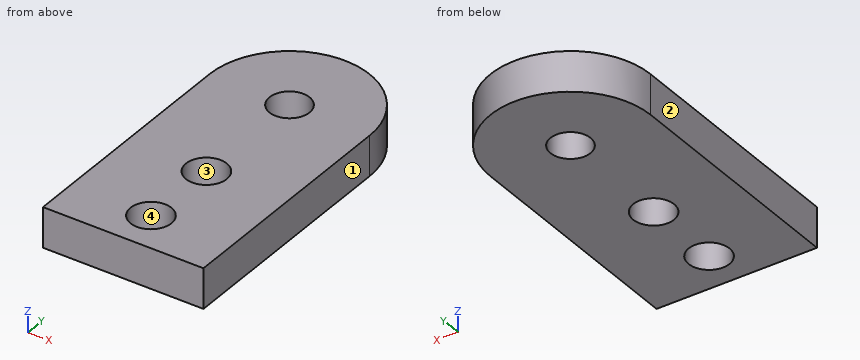
from build123d import *

# Parameters (mm, degrees)
SKETCH1_R           = 2.55
BOSS_EXTRUDE1_DEPTH = 5
SKETCH2_R           = 2.5
CUT_EXTRUDE1_DEPTH  = 5


with BuildPart() as part:
    # Sketch1 → Boss-Extrude1 (new body)
    with BuildSketch(Plane.XY):
        with BuildLine():
            Line((-10, 0), (-10, -30))
            Line((-10, -30), (10, -30))
            Line((10, -30), (10, 0))
            ThreePointArc((10, 0), (0, 10), (-10, 0))
        make_face()
        with Locations((0, -25)):
            Circle(SKETCH1_R, mode=Mode.SUBTRACT)
        with Locations((0, -15)):
            Circle(SKETCH1_R, mode=Mode.SUBTRACT)
    extrude(amount=BOSS_EXTRUDE1_DEPTH)

    # Sketch2 → Cut-Extrude1 (cut)
    with BuildSketch(Plane.XY.offset(5)):
        Circle(SKETCH2_R)
    extrude(amount=-CUT_EXTRUDE1_DEPTH, mode=Mode.SUBTRACT)


solid = part.part
The model under review builds one solid part; all positions refer to its coordinate system, in mm. Face numbers are marked on the shaded views. Give positions to 0.01 mm unless a question says otherwise; leave off trailing zeros. Order: outer loops, then holes, each group sorted by start corner. A loop starts at its lowest first (then second) coordinate and runs counter-clockwise, first axis right, second up. Notation, with made-up numbers: M 2.25,37 L 36.25,37 A17 ccw 36.25,59 Z; hole C 66.5,40 d11. An arc over 180 degrees is marked long. One line per question, with ' | ' between items. Start each with the question number.
1) Mouldability with a two-part tool opening along X and no side actions: class the marked faces 1, 2, 3 and 4 as pulls with the +X half, pulls with the -X half, needs draft (parallel to the pull), parting line crosses it, or undercut.
2) Consider section B-B, the plane y = -15. Give the boundary of the cut face in (x, z), then the cut area to 3 significant figures.
3) Consider section D-D, the plane x = 2. Give the boundary of the cut face in (y, z).
4) Consider section A-A, the plane z = 3.75. Give the boundary of the cut face in (x, y).
5) Consider section C-C, the plane x = 0. Give the boundary of the cut face in (y, z), then the cut area to 3 significant figures.
6) Wall thickness on L1, parallel to Y at x = 0, z = 3.1; L2, parallel to Y at x = 0.75, z = 4.4; L3, parallel to X at y = -2, z = 3.2: over which ranges is each line inside the solid? List them lowest first. Write a range as from..to.
Found:
1) face 1: pulls with the +X half | face 2: pulls with the -X half | face 3: undercut | face 4: undercut
2) outline: M -10,0 L -2.55,0 L -2.55,5 L -10,5 Z; M 2.55,0 L 10,0 L 10,5 L 2.55,5 Z | area: 74.5 mm²
3) outline: M -30,0 L -26.58,0 L -26.58,5 L -30,5 Z; M -23.42,0 L -16.58,0 L -16.58,5 L -23.42,5 Z; M -13.42,0 L -1.5,0 L -1.5,5 L -13.42,5 Z; M 1.5,0 L 9.8,0 L 9.8,5 L 1.5,5 Z
4) outline: M -10,-30 L 10,-30 L 10,0 A10 ccw -10,0 Z; hole C 0,-25 d5.1; hole C 0,-15 d5.1; hole C 0,0 d5
5) outline: M -30,0 L -27.55,0 L -27.55,5 L -30,5 Z; M -22.45,0 L -17.55,0 L -17.55,5 L -22.45,5 Z; M -12.45,0 L -2.5,0 L -2.5,5 L -12.45,5 Z; M 2.5,0 L 10,0 L 10,5 L 2.5,5 Z | area: 124 mm²
6) L1: y = -30..-27.55, -22.45..-17.55, -12.45..-2.5, 2.5..10 | L2: y = -30..-27.44, -22.56..-17.44, -12.56..-2.38, 2.38..9.97 | L3: x = -10..-1.5, 1.5..10
